Build history of the part. All positions in model axes, mm. A direction names the side the tool comes from. Coordinates: 2 decimals unless noted, no trailing zeros. Loops run counter-clockwise (first coordinate to the right, second up) from the corner with the lowest first, then second, coordinate; pieces in that order, holes last.
(1) Slice it at A-A (z = -53). Give the cut face in (x, y).
(2) Tool access for faces 1 (the face through (374, 4, -34)), 2 (the face through (374, 32, 0)): list every direction of +Z, -Z, +X, -X, +Y, -Y with a clear straight run to the whole face (end or side of a thin tool).
(3) Slice it at B-B (x = 400). Give the cut face in (y, z).
(4) Wall check: L1, parallel to Z at x = 635, y = 1.6; L2, parallel to Y at x = 75, z = -1; L3, parallel to Z at x = 587.5, y = 53. Give the ranges that are in metal, low to high.
(5) Flat gauge pins, fed straight in: P1, Ø11.5, axis at x = 25, y = 35, coming from the -Z side; P2, Ø8, axis at x = 642.5, z = -13, coming from the +Y side. Where does each tip first touch, or does it go through?
from build123d import *

# Parameters (mm, degrees)
EXTRUDE_1_DEPTH     = 758
SKETCH_2_R          = 5
CUT_EXTRUDE_1_DEPTH = 10
SKETCH_3_R          = 5
CUT_EXTRUDE_2_DEPTH = 10


with BuildPart() as part:
    # Эскиз1 → Вытянуть-Тонкостенный1 (new body)
    with BuildSketch(Plane(origin=(0, 0, 0), x_dir=(0, 0, -1), z_dir=(1, 0, 0))):
        Polygon((65, 0), (0, 0), (0, 65), (4, 65), (4, 4), (65, 4), align=None)
    extrude(amount=EXTRUDE_1_DEPTH)

    # Эскиз2 → Вырез-Вытянуть1 (cut)
    with BuildSketch(Plane.XY):
        with Locations((25, 35)):
            Circle(SKETCH_2_R)
        with Locations((75, 35)):
            Circle(SKETCH_2_R)
        with Locations((735, 35)):
            Circle(SKETCH_2_R)
        with Locations((635, 35)):
            Circle(SKETCH_2_R)
    extrude(amount=-CUT_EXTRUDE_1_DEPTH, mode=Mode.SUBTRACT)

    # Эскиз3 → Вырез-Вытянуть2 (cut)
    with BuildSketch(Plane.XZ):
        with Locations((25, -35)):
            Circle(SKETCH_3_R)
        with Locations((75, -35)):
            Circle(SKETCH_3_R)
        with Locations((735, -35)):
            Circle(SKETCH_3_R)
        with Locations((635, -35)):
            Circle(SKETCH_3_R)
    extrude(amount=-CUT_EXTRUDE_2_DEPTH, mode=Mode.SUBTRACT)


solid = part.part
Response values:
1. outline: (0, 0) - (758, 0) - (758, 4) - (0, 4) - close
2. face 1: -Z, +X, -X, +Y
2. face 2: +Z, +X, -X, +Y, -Y
3. outline: (0, -65) - (4, -65) - (4, -4) - (65, -4) - (65, 0) - (0, 0) - close
4. L1: z = -65 to -40, -30 to 0
4. L2: y = 0 to 30, 40 to 65
4. L3: z = -4 to 0
5. P1: stops at z = -4
5. P2: stops at y = 4
